from build123d import *

# Parameters (mm, degrees)
SKETCH1_W           = 30
SKETCH1_H           = 50
SKETCH1_R           = 1.5
BOSS_EXTRUDE1_DEPTH = 10
SKETCH3_R           = 2
CUT_EXTRUDE1_DEPTH  = 10


with BuildPart() as part:
    # Sketch1 → Boss-Extrude1 (new body)
    with BuildSketch(Plane.XY):
        Rectangle(SKETCH1_W, SKETCH1_H)
        with Locations((-8, 19)):
            Circle(SKETCH1_R, mode=Mode.SUBTRACT)
        with Locations(Location((8, 19, 0), (0, 0, 180))):
            Circle(SKETCH1_R, mode=Mode.SUBTRACT)
        with Locations((8, -19)):
            Circle(SKETCH1_R, mode=Mode.SUBTRACT)
        with Locations(Location((-8, -19, 0), (0, 0, 180))):
            Circle(SKETCH1_R, mode=Mode.SUBTRACT)
    extrude(amount=BOSS_EXTRUDE1_DEPTH)

    # Sketch3 → Cut-Extrude1 (cut)
    with BuildSketch(Plane.ZY.offset(15)):
        with Locations(Location((5, 12.5, 0), (0, 0, 270))):
            Circle(SKETCH3_R)
        with Locations(Location((5, -12.5, 0), (0, 0, 90))):
            Circle(SKETCH3_R)
    extrude(amount=-CUT_EXTRUDE1_DEPTH, mode=Mode.SUBTRACT)


solid = part.part
The listing builds one solid part. Answer for the finished solid, in the listing's coordinates (mm). A direction names the side the tool comes from. Give positions to 0.01 mm unless a question says otherwise; leave off trailing zeros. Write each loop counter-clockwise with the first axis right and the second up, starting at its lowest first coordinate (ties: lowest second). Pieces come first, ordered by that corner, then holes.
Item 1: Section A-A, the plane y = 19 is taken. Write down the section's boundary in (x, z), plus the area to 3 significant figures.
Item 2: Determine the mould class of faces 1 (the flat face through (0, 0, 10)), 2 (the cylindrical face through (-10.07, 14.498, 5.088)), 3 (the flat face through (-5, 13, 5)), 4 (the flat face through (15, 0, 5)) for opening direction Z: released by +Z, released by -Z, zero draft, split by the parting line, or undercut.
Item 3: Find the intervals of material crossed by line 1 along Y through (x, z) = (8, 2.5); line 2 along Y through (x, z) = (-8.5, 2.5); line 3 along X through (y, z) = (-18, 7.75), in increasing order.
Item 4: Which of the six approach directions +Z, -Z, +X, -X, +Y, -Y give full straight-line access (tool end or side, diameter ignored) to faces 5 (the cylindrical face through (-10.1, -14.1, 6.2)), 6 (the cylindrical face through (6.89, -17.99, 4.93))?
Item 5: Section D-D, the plane y = -20 is taken. Write down the section's boundary in (x, z), plus the area to 3 significant figures.
Item 6: Section B-B, the plane z = 1 is taken. Write down the section's boundary in (x, y).
Item 7: A flat-ended cylindrical pin translates along its axis: P1, Ø1.2, axis at y = 13, z = 4, coming from the -X side. Find the tip coordinate at first contact, or state that the pin passes through.
Item 8: Section C-C, the plane y = -12.5 is taken. Write down the section's boundary in (x, z), plus the area to 3 significant figures.
Completed:
1. outline: (-15, 0) - (-9.5, 0) - (-9.5, 10) - (-15, 10) - close; (-6.5, 0) - (6.5, 0) - (6.5, 10) - (-6.5, 10) - close; (9.5, 0) - (15, 0) - (15, 10) - (9.5, 10) - close
1. area: 240 mm2
2. face 1: released by +Z
2. face 2: undercut
2. face 3: undercut
2. face 4: zero draft
3. line 1: y = -25 to -20.5, -17.5 to 17.5, 20.5 to 25
3. line 2: y = -25 to -20.41, -17.59 to 17.59, 20.41 to 25
3. line 3: x = -15 to -9.12, -6.88 to 6.88, 9.12 to 15
4. face 5: -X
4. face 6: +Z, -Z
5. outline: (-15, 0) - (-9.12, 0) - (-9.12, 10) - (-15, 10) - close; (-6.88, 0) - (6.88, 0) - (6.88, 10) - (-6.88, 10) - close; (9.12, 0) - (15, 0) - (15, 10) - (9.12, 10) - close
5. area: 255 mm2
6. outline: (-15, -25) - (15, -25) - (15, 25) - (-15, 25) - close; hole circle Ø3 at (-8, -19); hole circle Ø3 at (-8, 19); hole circle Ø3 at (8, -19); hole circle Ø3 at (8, 19)
7. P1: stops at x = -5
8. outline: (-15, 0) - (15, 0) - (15, 10) - (-15, 10) - (-15, 7) - (-5, 7) - (-5, 3) - (-15, 3) - close
8. area: 260 mm2
